For this review, take the finished solid that the model builds, in its own axes (mm). Face numbers are marked on the shaded views. A direction names the side the tool comes from. Coordinates: 2 decimals unless noted, no trailing zeros. Order: outer loops, then holes, each group sorted by start corner. A loop starts at its lowest first (then second) coordinate and runs counter-clockwise, first axis right, second up. Notation, with made-up numbers: (84.5, 15) -> (113.5, 15) arc R23 ccw to (113.5, 44) -> close; hole circle Ø4 at (34, -1). An arc over 180 degrees is marked (long way). Write item = value, one per line. Start each with the question number.
1) Consider section A-A on x = 30. Give the boundary of the cut face in (y, z), and give its area (3 significant figures).
2) Consider section B-B on y = 85. Give the boundary of the cut face in (x, z).
3) Machinability: for the marked faces 1 and 2, which of the approach directions +Z, -Z, +X, -X, +Y, -Y give a long, thin tool a straight path to every point of the face, cutting with its end or side? Answer none if there is none.
4) Insertion check: pin 1 Ø23 at (x, y) = (33, 111.5) entering from +Z; pin 2 Ø3.5 at (x, z) = (38, 5.5) entering from -Y; pin 3 Ø2 at (x, z) = (80, 7) entering from +Y. Each pin has a flat end and moves straight along its axis. Give the tip position at first contact, or say it passes through.
5) Consider section C-C on y = 118. Give the boundary of the cut face in (x, z), and give its area (4 significant figures).
6) Consider section D-D on x = 43. Give the boundary of the cut face in (y, z), and give its area (3 significant figures).
7) Wall thickness on probe 1 along Z at (x, y) = (9, 101.5); probe 2 along X at (y, z) = (130, 3.5); probe 3 along X at (y, z) = (86, 4.25): over which ranges is each line inside the solid? List them lowest first. Write a range as [from, to].
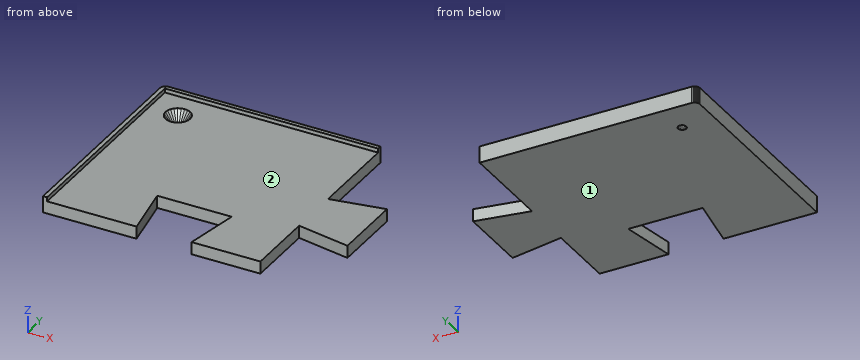
from build123d import *

# Parameters (mm, degrees)
BOSS_EXTRUDE1_DEPTH = 6
SKETCH2_W           = 4.5
SKETCH2_H           = 48.026539614
BOSS_EXTRUDE2_DEPTH = 19.5
SKETCH3_W           = 1.5
SKETCH3_H           = 77.5
CUT_EXTRUDE1_DEPTH  = 77.5
SKETCH4_W           = 27.053079228
SKETCH4_H           = 20
CUT_EXTRUDE2_DEPTH  = 184.532694635
SKETCH5_W           = 19.5
SKETCH5_H           = 21.973460386
CUT_EXTRUDE3_DEPTH  = 184.532694635
CUT_EXTRUDE4_DEPTH  = 4.5
CUT_EXTRUDE4_TAPER  = -33.463237765
DRAFT1_ANGLE        = -10
DRAFT2_ANGLE        = -10.251039049


with BuildPart() as part:
    # Sketch1 → Boss-Extrude1 (new body)
    with BuildSketch(Plane.XY.offset(9.15)):
        Polygon((-2, 77), (77, 77), (77, 156), (0, 156), (-0.51763809, 155.931851653), (-0.765366865, 155.847759065), (-1, 155.732050808), (-1.217522858, 155.586706681), (-1.414213562, 155.414213562), (-1.586706681, 155.217522858), (-1.732050808, 155), (-1.847759065, 154.765366865), (-1.931851653, 154.51763809), (-2, 154), align=None)
    extrude(amount=-BOSS_EXTRUDE1_DEPTH)

    # Sketch2 → Boss-Extrude2 (add)
    with BuildSketch(Plane(origin=(77, 0, 0), x_dir=(0, 0, -1), z_dir=(1, 0, 0))):
        with Locations((-5.4, 101.013269807)):
            Rectangle(SKETCH2_W, SKETCH2_H)
    extrude(amount=BOSS_EXTRUDE2_DEPTH)

    # Sketch3 → Cut-Extrude1 (cut)
    with BuildSketch(Plane(origin=(77, 0, 0), x_dir=(0, 0, -1), z_dir=(1, 0, 0))):
        with Locations((-8.4, 115.75)):
            Rectangle(SKETCH3_W, SKETCH3_H)
    extrude(amount=-CUT_EXTRUDE1_DEPTH, mode=Mode.SUBTRACT)

    # Sketch4 → Cut-Extrude2 (cut, through all)
    with BuildSketch(Plane(origin=(0, 0, 3.15), x_dir=(-1, 0, 0), z_dir=(0, 0, -1))):
        with Locations((-42, 87)):
            Rectangle(SKETCH4_W, SKETCH4_H)
    extrude(amount=-CUT_EXTRUDE2_DEPTH, mode=Mode.SUBTRACT)

    # Sketch5 → Cut-Extrude3 (cut, through all)
    with BuildSketch(Plane(origin=(0, 0, 3.15), x_dir=(-1, 0, 0), z_dir=(0, 0, -1))):
        with Locations((-86.75, 87.986730193)):
            Rectangle(SKETCH5_W, SKETCH5_H)
    extrude(amount=-CUT_EXTRUDE3_DEPTH, mode=Mode.SUBTRACT)

    # Sketch6 → Cut-Extrude4 (cut)
    with BuildSketch(Plane(origin=(0, 0, 3.15), x_dir=(-1, 0, 0), z_dir=(0, 0, -1))):
        Polygon((-11.060660172, 142.939339828), (-10.75, 142.700961894), (-10.388228568, 142.551111261), (-10, 142.5), (-9.611771432, 142.551111261), (-9.25, 142.700961894), (-8.939339828, 142.939339828), (-8.700961894, 143.25), (-8.551111261, 143.611771432), (-8.5, 144), (-8.551111261, 144.388228568), (-8.700961894, 144.75), (-8.939339828, 145.060660172), (-9.25, 145.299038106), (-9.611771432, 145.448888739), (-10, 145.5), (-10.388228568, 145.448888739), (-10.75, 145.299038106), (-11.060660172, 145.060660172), (-11.299038106, 144.75), (-11.448888739, 144.388228568), (-11.5, 144), (-11.448888739, 143.611771432), (-11.299038106, 143.25), align=None)
    extrude(amount=-CUT_EXTRUDE4_DEPTH, taper=CUT_EXTRUDE4_TAPER, mode=Mode.SUBTRACT)

    # Draft1
    draft1_faces = [part.faces().sort_by_distance(p)[0] for p in [
        (55.526539614, 87, 5.4),
        (28.473460386, 87, 5.4),
    ]]
    draft(draft1_faces, Plane(origin=(28.473460386, 97, 9.15), x_dir=(-1, 0, 0), z_dir=(0, -1, 0)), DRAFT1_ANGLE)

    # Draft2
    draft2_faces = [part.faces().sort_by_distance(p)[0] for p in [
        (86.75, 98.973460386, 5.4),
        (86.75, 125.026539614, 5.4),
    ]]
    draft(draft2_faces, Plane.YZ.offset(96.5), DRAFT2_ANGLE)


solid = part.part
Answer sheet:
q1.outline = (77, 3.15) -> (88.34, 3.15) -> (88.34, 7.65) -> (77, 7.65) -> close; (97, 3.15) -> (156, 3.15) -> (156, 9.15) -> (154.5, 9.15) -> (154.5, 7.65) -> (97, 7.65) -> close
q1.area = 319 mm2
q2.outline = (-2, 3.15) -> (30.59, 3.15) -> (30.59, 7.65) -> (-0.5, 7.65) -> (-0.5, 9.15) -> (-2, 9.15) -> close; (53.41, 3.15) -> (77, 3.15) -> (77, 7.65) -> (53.41, 7.65) -> close
q3.face_1 = -Z, +X, -X, +Y, -Y
q3.face_2 = +Z, +X, -Y
q4.pin_1 = 7.65
q4.pin_2 = 97
q4.pin_3 = 122.22
q5.outline = (-2, 3.15) -> (96.5, 3.15) -> (96.5, 7.65) -> (-0.5, 7.65) -> (-0.5, 9.15) -> (-2, 9.15) -> close
q5.area = 445.5 mm2
q6.outline = (97, 3.15) -> (156, 3.15) -> (156, 9.15) -> (154.5, 9.15) -> (154.5, 7.65) -> (97, 7.65) -> close
q6.area = 268 mm2
q7.probe_1 = [3.15, 7.65]
q7.probe_2 = [-2, 77]
q7.probe_3 = [-2, 30.41], [53.59, 77]
